Read the model definition and answer for the solid it produces. Units are mm, in the model's axes. Round coordinates to 2 decimals unless told otherwise and drop trailing zeros. Order: outer loops, then holes, each group sorted by start corner. A loop starts at its lowest first (then second) coordinate and runs counter-clockwise, first axis right, second up.
from build123d import *

# Parameters (mm, degrees)
SKETCH1_R           = 10
SKETCH1_R_2         = 9
BOSS_EXTRUDE1_DEPTH = 116
SKETCH3_R           = 2
CUT_EXTRUDE2_DEPTH  = 21


with BuildPart() as part:
    # Sketch1 → Boss-Extrude1 (new body)
    with BuildSketch(Plane(origin=(0, 0, 0), x_dir=(1, 0, 0), z_dir=(0, 1, 0))):
        Circle(SKETCH1_R)
        Circle(SKETCH1_R_2, mode=Mode.SUBTRACT)
    extrude(amount=BOSS_EXTRUDE1_DEPTH)

    # Sketch3 → Cut-Extrude2 (cut, through all)
    with BuildSketch(Plane(origin=(10, 0, 0), x_dir=(0, 0, -1), z_dir=(1, 0, 0))):
        with Locations((0, 103.5)):
            Circle(SKETCH3_R)
        with Locations((0, 12.5)):
            Circle(SKETCH3_R)
    extrude(amount=-CUT_EXTRUDE2_DEPTH, mode=Mode.SUBTRACT)


solid = part.part
Q1. Straight lines are drawn through the part: probe 1 along Y at (x, z) = (-9.3, 0); probe 2 along Z at (x, y) = (-3.25, 82); probe 3 along X at (y, z) = (38.5, -2.5). For each, find the intervals that lie inside material, in ascending order.
Outcome:
probe 1: y = 0 to 10.5, 14.5 to 101.5, 105.5 to 116
probe 2: z = -9.46 to -8.39, 8.39 to 9.46
probe 3: x = -9.68 to -8.65, 8.65 to 9.68
Q2. Flat-ended cylindrical pins translate along their axes: pin 1 (12 mm diameter, centred on x = -3.5, z = -2, fed in from +Y); pin 2 (12 mm diameter, centred on x = -6.5, y = 90.5, fed in from +Z); pin 3 (6 mm diameter, centred on x = 7.5, y = 77.5, fed in from -Z); pin 4 (2 mm diameter, centred on y = 30, z = 7, fed in from +X). Find the tip coordinate at first contact, or state that the pin passes through.
Outcome:
pin 1: stops at y = 116
pin 2: stops at z = 9.99
pin 3: stops at z = -8.93
pin 4: stops at x = 8
Q3. A cutting plane is placed at D-D, the plane y = 35.5. Give the vertices of the cut face in (x, z), plus the area to 3 significant figures.
Outcome:
outline: circle Ø20 at (0, 0); hole circle Ø18 at (0, 0)
area: 59.7 mm2
Q4. A cutting plane is placed at A-A, the plane z = 0. Give the vertices of the cut face in (x, y).
Outcome:
outline: (-10, 0) - (-9, 0) - (-9, 10.5) - (-10, 10.5) - close; (-10, 14.5) - (-9, 14.5) - (-9, 101.5) - (-10, 101.5) - close; (-10, 105.5) - (-9, 105.5) - (-9, 116) - (-10, 116) - close; (9, 0) - (10, 0) - (10, 10.5) - (9, 10.5) - close; (9, 14.5) - (10, 14.5) - (10, 101.5) - (9, 101.5) - close; (9, 105.5) - (10, 105.5) - (10, 116) - (9, 116) - close
Q5. A cutting plane is placed at C-C, the plane y = 103.5. Give the vertices of the cut face in (x, z).
Outcome:
outline: (-9.8, -2) arc R10 ccw to (9.8, -2) - (8.77, -2) arc R9 cw to (-8.77, -2) - close; (-9.8, 2) - (-8.77, 2) arc R9 cw to (8.77, 2) - (9.8, 2) arc R10 ccw to start
Q6. For a pull along X with two mould halves and no side action, classify faces 1 (the face through (-9, 116, -2)), 2 (the face through (-2.17, 57.19, 9.76)), 3 (the face through (-1.172, 57.188, -8.923)) as released by +X, released by -X, zero draft, split by the parting line, or undercut.
Outcome:
face 1: zero draft
face 2: split by the parting line
face 3: undercut
Q7. A cutting plane is placed at B-B, the plane x = -6. Give the vertices of the cut face in (y, z).
Outcome:
outline: (0, -8) - (116, -8) - (116, -6.71) - (0, -6.71) - close; (0, 6.71) - (116, 6.71) - (116, 8) - (0, 8) - close
